CAD build for the part. Positions are in the model's coordinates, mm. Give positions to 0.01 mm unless a question says otherwise; leave off trailing zeros.
Item 1: Wall check: L1, parallel to Y at x = -51.5, z = -13.5; L2, parallel to Y at x = -129, z = 5; L3, parallel to Z at x = -62, y = 129. Give the ranges that are in metal, low to high.
Item 2: Two-plate mould, pull along Z, no slides. Class faces 1 (the flat face through (-127.5, 87, -14.1)), 2 (the cylindrical face through (-23.149, 94.106, 23.323)), 3 (the flat face through (-64.338, 142.751, -21.337)): released by +Z, released by -Z, zero draft, split by the parting line, or undercut.
Item 3: Flat gauge pins, fed straight in: P1, Ø12, axis at x = -103.5, y = 101, coming from the +Z side; P2, Ø8, axis at y = 160.5, z = -16.5, coming from the +X side; P3, Ø12, axis at y = 166.5, z = 15.5, coming from the -X side. Where does each tip first touch, or does it go through?
```python
from build123d import *

# Parameters (mm, degrees)
SKETCH2_R             = 32.184938318
BOSS_EXTRUDE1_DEPTH   = 78
SKETCH3_R             = 44.452761075
BOSS_EXTRUDE2_DEPTH   = 48
BODY_MOVE_COPY2_ANGLE = 94.867085016


with BuildPart() as part:
    # Sketch2 → Boss-Extrude1 (new body)
    with BuildSketch(Plane(origin=(0, 0, 0), x_dir=(1, 0, 0), z_dir=(0, 1, 0))):
        Circle(SKETCH2_R)
    extrude(amount=BOSS_EXTRUDE1_DEPTH)

    # Sketch3 → Boss-Extrude2 (add)
    with BuildSketch(Plane(origin=(0, 78, 0), x_dir=(1, 0, 0), z_dir=(0, 1, 0))):
        Circle(SKETCH3_R)
    extrude(amount=BOSS_EXTRUDE2_DEPTH)


with BuildPart() as part_1:
    # Body-Move/Copy1: moved
    add(part.part.moved(Location((-72.960744445, 52.218831428, 0))))


with BuildPart() as part_2:
    # Body-Move/Copy2: moved
    add(part_1.part.moved(Location((0, 0, 0))).rotate(Axis((-95.551423715, 86.931599726, 17.334437881), (0.562837469, 0.704764727, -0.43188038)), BODY_MOVE_COPY2_ANGLE))


solid = part_2.part
```
The answers:
1. L1: y = 94.52 to 169.32
1. L2: y = 80.15 to 117.18
1. L3: z = -28.45 to 48.92
2. face 1: released by -Z
2. face 2: split by the parting line
2. face 3: undercut
3. P1: stops at z = 26.5
3. P2: stops at x = -16.86
3. P3: stops at x = -79.56
